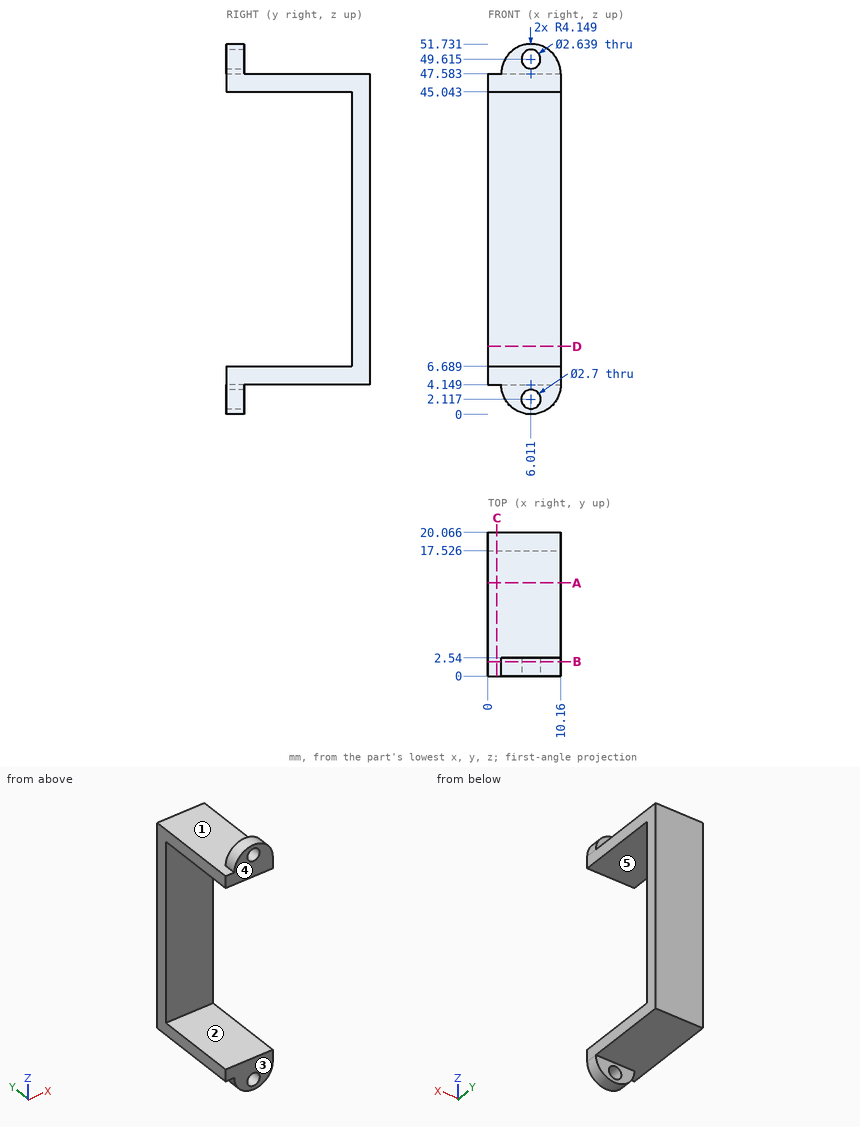
Geometry: see drawing. Coordinates: mm, zero at the bounding-box minimum. A direction names the side the tool comes from. Round coordinates to 2 decimals unless told otherwise and drop trailing zeros. Order: outer loops, then holes, each group sorted by start corner. A loop starts at its lowest first (then second) coordinate and runs counter-clockwise, first axis right, second up. Notation, with made-up numbers: (67.5, 78) - (106.5, 78) arc R21 ccw to (106.5, 101) - close; hole circle Ø11 at (-4, 2). An arc over 180 degrees is marked (long way). Use a Markdown table: item, result. Add a question column.
1. Mould query, pull axis Z, two halves, no side actions, for the marked faces 1, 2 and 3. Classes: +Z half, -Z half, draft (parallel to the pull), parting line (faces both ways), or undercut.
2. Section query C-C (x = 1.25). Return the cut outline in (y, z).
3. Section query A-A (y = 13). Return the cut outline in (x, z).
4. First-contact query: pin 1 (3 mm diameter, centred on x = 4, y = 14.5, fed in from +Z); pin 2 (3.5 mm diameter, centred on x = 4.5, z = 48.5, fed in from +Y); pin 3 (3.5 mm diameter, centred on x = 6.01, z = 49.61, fed in from +Y); pin 4 (1 mm diameter, centred on x = 4, y = 17, fed in from -Z). Flat tips, straight axial feed; report the tip coordinate or a pass-through.
5. Set-up query: the marked faces 4 and 5. Return all of +Z, -Z, +X, -X, +Y, -Y with unobstructed straight access to the full face (end or side cutting, diameter ignored); none if empty.
6. Line query: probe 1 along Z at (x, y) = (1.75, 3.5); probe 2 along Z at (x, y) = (5, 2.5) (1 decimal); probe 3 along Y at (x, z) = (9.25, 23.5). Output: solid intervals per line, ascending.
7. Section query D-D (z = 9.5). Return the cut outline in (x, y).
8. Section query B-B (y = 2). Give the number of separate pieces and of enclosed holes in the cut face.
Derived:
| question | item | result |
|---|---|---|
| 1 | face 1 | +Z half |
| 1 | face 2 | undercut |
| 1 | face 3 | draft |
| 2 | outline | (0, 4.15) - (20.07, 4.15) - (20.07, 47.58) - (0, 47.58) - (0, 45.04) - (17.53, 45.04) - (17.53, 6.69) - (0, 6.69) - close |
| 3 | outline | (0, 4.15) - (10.16, 4.15) - (10.16, 6.69) - (0, 6.69) - close; (0, 45.04) - (10.16, 45.04) - (10.16, 47.58) - (0, 47.58) - close |
| 4 | pin 1 | z = 47.58 |
| 4 | pin 2 | y = 20.07 |
| 4 | pin 3 | y = 2.54 |
| 4 | pin 4 | z = 4.15 |
| 5 | face 4 | +Z, -Z, +X, -X, -Y |
| 5 | face 5 | +X, -X, -Y |
| 6 | probe 1 | 4.15 to 6.69, 45.04 to 47.58 |
| 6 | probe 2 | 0.1 to 1.2, 3 to 6.7, 45 to 48.8, 50.5 to 51.6 |
| 6 | probe 3 | 17.53 to 20.07 |
| 7 | outline | (0, 17.53) - (10.16, 17.53) - (10.16, 20.07) - (0, 20.07) - close |
| 8 | separate pieces | 2 |
| 8 | enclosed holes | 2 |
